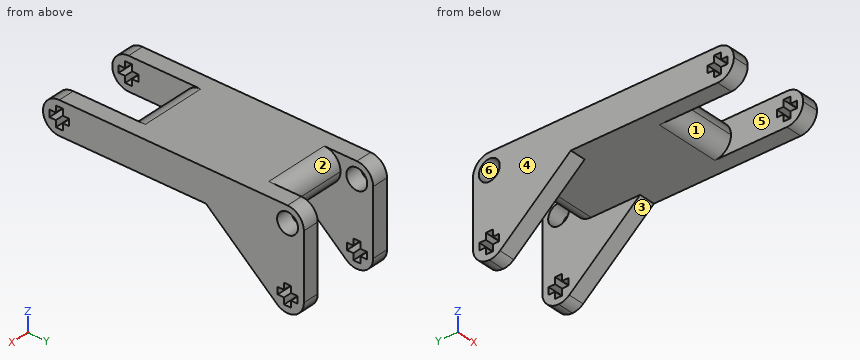
from build123d import *

# Parameters (mm, degrees)
F1_DEPTH = 7.9375
F2_R     = 3.96874
F3_W     = 3.96875
F3_H     = 23.8125
F4_DEPTH = 15.875
F5_W     = 1.56845
F5_H     = 1.6891
F5_W_2   = 1.6891
F5_H_2   = 1.56845
F5_R     = 2.54
F6_DEPTH = 23.8125


# Not quite as in the source:
# - a fillet or chamfer is up to 0.001 mm smaller than in the source, because OpenCascade refuses the exact size


with BuildPart() as f1:
    # F0 (on Top) → F1 (new body)
    with BuildSketch(Plane.XY):
        Polygon((0, 63.5), (0, 0), (3.96875, 0), (3.96875, 17.5562514), (19.84375, 17.5562514), (19.84375, 0), (23.8125, 0), (23.8125, 63.5), (19.84375, 63.5), (19.84375, 55.5625), (3.96875, 55.5625), (3.96875, 63.5), align=None)
    extrude(amount=F1_DEPTH)

    # F2 (radius 3.96875 in the source; OpenCascade refuses exactly that, so slightly less here)
    f2_edges = [f1.edges().sort_by_distance(p)[0] for p in [
        (11.90625, 55.5625, 7.9375),
        (11.90625, 55.5625, 0),
        (1.984375, 63.5, 7.9375),
        (21.828125, 63.5, 7.9375),
        (1.984375, 0, 7.9375),
        (1.984375, 0, 0),
        (21.828125, 0, 7.9375),
        (21.828125, 0, 0),
        (11.90625, 17.556251, 7.9375),
        (11.90625, 17.556251, 0),
    ]]
    fillet(f2_edges, radius=F2_R)

    # F3 (on face) → F4 (join)
    with BuildSketch(Plane(origin=(0, 0, 0), x_dir=(1, 0, 0), z_dir=(0, 0, -1))):
        with Locations((21.828125, -51.59375)):
            Rectangle(F3_W, F3_H)
        with Locations((1.984375, -51.59375)):
            Rectangle(F3_W, F3_H)
    extrude(amount=F4_DEPTH)

    # F5 (on face) → F6 (cut, through all)
    with BuildSketch(Plane(origin=(0, 0, 0), x_dir=(0, -1, 0), z_dir=(-1, 0, 0))):
        with Locations((-5.597525, 3.96875)):
            Rectangle(F5_W, F5_H)
        with Locations((-3.96875, 3.96875)):
            Rectangle(F5_W_2, F5_H)
        with Locations((-3.96875, 2.339975)):
            Rectangle(F5_W_2, F5_H_2)
        with Locations((-2.339975, 3.96875)):
            Rectangle(F5_W, F5_H)
        with Locations((-3.96875, 5.597525)):
            Rectangle(F5_W_2, F5_H_2)
        with BuildLine():
            Line((-63.5, -15.875), (-59.53125, -15.875))
            ThreePointArc((-59.53125, -15.875), (-62.3375800378, -14.7125800378), (-63.5, -11.90625))
            Line((-63.5, -11.90625), (-63.5, -15.875))
        make_face()
        with BuildLine():
            Line((-59.53125, -15.875), (-39.6875, -15.875))
            Line((-39.6875, -15.875), (-39.6875, 0))
            Line((-39.6875, 0), (-56.935957382, -14.9088210299))
            ThreePointArc((-56.935957382, -14.9088210299), (-58.146597916, -15.6256202651), (-59.53125, -15.875))
        make_face()
        with Locations((-57.902475, -11.90625)):
            Rectangle(F5_W, F5_H)
        with Locations((-59.53125, -11.90625)):
            Rectangle(F5_W_2, F5_H)
        with Locations((-59.53125, -10.277475)):
            Rectangle(F5_W_2, F5_H_2)
        with Locations((-61.160025, -11.90625)):
            Rectangle(F5_W, F5_H)
        with Locations((-59.53125, -13.535025)):
            Rectangle(F5_W_2, F5_H_2)
        with Locations((-59.53125, 3.96875)):
            Circle(F5_R)
    extrude(amount=-F6_DEPTH, mode=Mode.SUBTRACT)


solid = f1.part
Source: CAD feature listing. Evaluate the final solid. Frame: model axes, mm. Face numbers are marked on the shaded views. A direction names the side the tool comes from. Round coordinates to 2 decimals unless told otherwise and drop trailing zeros. Loops run counter-clockwise (first coordinate to the right, second up) from the corner with the lowest first, then second, coordinate; pieces in that order, holes last. Notation, with made-up numbers: (43, 1.5) - (74, 1.5) arc R18 ccw to (74, 6.5) - close; hole circle Ø3 at (13, 43). An arc over 180 degrees is marked (long way). Write item = value, one per line. Start each with the question number.
Item 1: Section query D-D on x = 22.75. Count the separate pieces of the cut face and the enclosed holes in it, plus the area to 3 significant figures.
Item 2: Mould query, pull axis X, two halves, no side actions, for the marked faces 4, 5 and 6. Classes: released by +X, released by -X, zero draft, split by the parting line, or undercut.
Item 3: Section query C-C on y = 32. Output: boundary loops of the cut face in (x, z), plus the area to 3 significant figures.
Item 4: Section query B-B on z = -8.75. Output: boundary loops of the cut face in (x, y).
Item 5: Material intervals for line 1 (Y direction, x = 22, z = 3.75); line 2 (Z direction, x = 22.5, y = 6); line 3 (X direction, y = 14, z = 1.75), sorted ascending.
Item 6: Reachability of the marked faces 1, 2 and 3 from +Z, -Z, +X, -X, +Y, -Y: full face, straight path, thin tool, end or side. Return the list, or none.
Item 7: First-contact query: pin 1 Ø0.8 at (x, y) = (22.5, 57.5) entering from -Z; pin 2 Ø3 at (x, z) = (19, 1) entering from -Y; pin 3 Ø8 at (x, z) = (17, -10) entering from -Y; pin 4 Ø10 at (y, z) = (9.5, -1) entering from -X. Flat tips, straight axial feed; report the tip coordinate or a pass-through.
Results list:
q1.separate_pieces = 1
q1.enclosed_holes = 3
q1.area = 675 mm²
q2.face_4 = released by -X
q2.face_5 = undercut
q2.face_6 = zero draft
q3.outline = (0, 0) - (23.81, 0) - (23.81, 7.94) - (0, 7.94) - close
q3.area = 189 mm²
q4.outline = (0, 49.81) - (3.97, 49.81) - (3.97, 63.5) - (0, 63.5) - close; (19.84, 49.81) - (23.81, 49.81) - (23.81, 63.5) - (19.84, 63.5) - close
q5.line_1 = 0.01 to 1.56, 6.38 to 57, 62.06 to 63.5
q5.line_2 = 0 to 3.12, 4.81 to 7.94
q5.line_3 = 0 to 3.97, 19.84 to 23.81
q6.face_1 = -Z, -Y
q6.face_2 = +Z, +Y
q6.face_3 = -Z, +X, -X, -Y
q7.pin_1 = -15.52
q7.pin_2 = 0.4
q7.pin_3 = 48
q7.pin_4 = 0
